Can you work these out from the model? Positions are in its coordinate system, mm. Coordinates: 2 decimals unless noted, no trailing zeros. Order: outer loops, then holes, each group sorted by start corner. A loop starts at its lowest first (then second) coordinate and runs counter-clockwise, first axis right, second up. Notation, with made-up numbers: (54, 1.5) -> (90, 1.5) arc R23 cw to (90, 38.5) -> close; hole circle Ø2 at (-13.5, 29.5). An arc over 180 degrees is marked (long way). Write item = value, one per line.
```python
from build123d import *

# Parameters (mm, degrees)
F0_R     = 14.732
F1_DEPTH = 3.175
F2_DEPTH = 2
F3_R     = 9.398
F4_DEPTH = 1.905
F6_R     = 0.635


# Not quite as in the source:
# - a fillet or chamfer that OpenCascade refuses, or shapes differently, is made with other operations: its cross-section is extruded or revolved along the edge and cut away or added


with BuildPart() as f1:
    # F0 (on Top) → F1 (new body)
    with BuildSketch(Plane.XY):
        Circle(F0_R)
        with BuildLine():
            ThreePointArc((-10.3772609868, 7.5395214312), (-6.4135, 11.1085078543), (-1.3407865983, 12.7567323519))
            Line((-1.3407865983, 12.7567323519), (-1.214689647, 11.557))
            Line((-1.214689647, 11.557), (1.214689647, 11.557))
            Line((1.214689647, 11.557), (1.3407865983, 12.7567323519))
            ThreePointArc((1.3407865983, 12.7567323519), (6.4135, 11.1085078543), (10.3772609868, 7.5395214312))
            Line((10.3772609868, 7.5395214312), (9.4013107681, 6.830452092))
            Line((9.4013107681, 6.830452092), (10.616000415, 4.726547908))
            Line((10.616000415, 4.726547908), (11.7180475852, 5.2172109207))
            ThreePointArc((11.7180475852, 5.2172109207), (12.827, 0), (11.7180475852, -5.2172109207))
            Line((11.7180475852, -5.2172109207), (10.616000415, -4.726547908))
            Line((10.616000415, -4.726547908), (9.4013107681, -6.830452092))
            Line((9.4013107681, -6.830452092), (10.3772609868, -7.5395214312))
            ThreePointArc((10.3772609868, -7.5395214312), (6.4135, -11.1085078543), (1.3407865983, -12.7567323519))
            Line((1.3407865983, -12.7567323519), (1.214689647, -11.557))
            Line((1.214689647, -11.557), (-1.214689647, -11.557))
            Line((-1.214689647, -11.557), (-1.3407865983, -12.7567323519))
            ThreePointArc((-1.3407865983, -12.7567323519), (-6.4135, -11.1085078543), (-10.3772609868, -7.5395214312))
            Line((-10.3772609868, -7.5395214312), (-9.4013107681, -6.830452092))
            Line((-9.4013107681, -6.830452092), (-10.616000415, -4.726547908))
            Line((-10.616000415, -4.726547908), (-11.7180475852, -5.2172109207))
            ThreePointArc((-11.7180475852, -5.2172109207), (-12.827, 0), (-11.7180475852, 5.2172109207))
            Line((-11.7180475852, 5.2172109207), (-10.616000415, 4.726547908))
            Line((-10.616000415, 4.726547908), (-9.4013107681, 6.830452092))
            Line((-9.4013107681, 6.830452092), (-10.3772609868, 7.5395214312))
        make_face(mode=Mode.SUBTRACT)
        with BuildLine():
            Line((-1.214689647, 11.557), (-1.3407865983, 12.7567323519))
            ThreePointArc((-1.3407865983, 12.7567323519), (-6.4135, 11.1085078543), (-10.3772609868, 7.5395214312))
            Line((-10.3772609868, 7.5395214312), (-9.4013107681, 6.830452092))
            Line((-9.4013107681, 6.830452092), (-10.616000415, 4.726547908))
            Line((-10.616000415, 4.726547908), (-11.7180475852, 5.2172109207))
            ThreePointArc((-11.7180475852, 5.2172109207), (-12.827, 0), (-11.7180475852, -5.2172109207))
            Line((-11.7180475852, -5.2172109207), (-10.616000415, -4.726547908))
            Line((-10.616000415, -4.726547908), (-9.4013107681, -6.830452092))
            Line((-9.4013107681, -6.830452092), (-10.3772609868, -7.5395214312))
            ThreePointArc((-10.3772609868, -7.5395214312), (-6.4135, -11.1085078543), (-1.3407865983, -12.7567323519))
            Line((-1.3407865983, -12.7567323519), (-1.214689647, -11.557))
            Line((-1.214689647, -11.557), (1.214689647, -11.557))
            Line((1.214689647, -11.557), (1.3407865983, -12.7567323519))
            ThreePointArc((1.3407865983, -12.7567323519), (6.4135, -11.1085078543), (10.3772609868, -7.5395214312))
            Line((10.3772609868, -7.5395214312), (9.4013107681, -6.830452092))
            Line((9.4013107681, -6.830452092), (10.616000415, -4.726547908))
            Line((10.616000415, -4.726547908), (11.7180475852, -5.2172109207))
            ThreePointArc((11.7180475852, -5.2172109207), (12.827, 0), (11.7180475852, 5.2172109207))
            Line((11.7180475852, 5.2172109207), (10.616000415, 4.726547908))
            Line((10.616000415, 4.726547908), (9.4013107681, 6.830452092))
            Line((9.4013107681, 6.830452092), (10.3772609868, 7.5395214312))
            ThreePointArc((10.3772609868, 7.5395214312), (6.4135, 11.1085078543), (1.3407865983, 12.7567323519))
            Line((1.3407865983, 12.7567323519), (1.214689647, 11.557))
            Line((1.214689647, 11.557), (-1.214689647, 11.557))
        make_face()
    extrude(amount=-F1_DEPTH)

    # F0 (on Top) → F2 (join)
    with BuildSketch(Plane.XY):
        Circle(F0_R)
        with BuildLine():
            ThreePointArc((-10.3772609868, 7.5395214312), (-6.4135, 11.1085078543), (-1.3407865983, 12.7567323519))
            Line((-1.3407865983, 12.7567323519), (-1.214689647, 11.557))
            Line((-1.214689647, 11.557), (1.214689647, 11.557))
            Line((1.214689647, 11.557), (1.3407865983, 12.7567323519))
            ThreePointArc((1.3407865983, 12.7567323519), (6.4135, 11.1085078543), (10.3772609868, 7.5395214312))
            Line((10.3772609868, 7.5395214312), (9.4013107681, 6.830452092))
            Line((9.4013107681, 6.830452092), (10.616000415, 4.726547908))
            Line((10.616000415, 4.726547908), (11.7180475852, 5.2172109207))
            ThreePointArc((11.7180475852, 5.2172109207), (12.827, 0), (11.7180475852, -5.2172109207))
            Line((11.7180475852, -5.2172109207), (10.616000415, -4.726547908))
            Line((10.616000415, -4.726547908), (9.4013107681, -6.830452092))
            Line((9.4013107681, -6.830452092), (10.3772609868, -7.5395214312))
            ThreePointArc((10.3772609868, -7.5395214312), (6.4135, -11.1085078543), (1.3407865983, -12.7567323519))
            Line((1.3407865983, -12.7567323519), (1.214689647, -11.557))
            Line((1.214689647, -11.557), (-1.214689647, -11.557))
            Line((-1.214689647, -11.557), (-1.3407865983, -12.7567323519))
            ThreePointArc((-1.3407865983, -12.7567323519), (-6.4135, -11.1085078543), (-10.3772609868, -7.5395214312))
            Line((-10.3772609868, -7.5395214312), (-9.4013107681, -6.830452092))
            Line((-9.4013107681, -6.830452092), (-10.616000415, -4.726547908))
            Line((-10.616000415, -4.726547908), (-11.7180475852, -5.2172109207))
            ThreePointArc((-11.7180475852, -5.2172109207), (-12.827, 0), (-11.7180475852, 5.2172109207))
            Line((-11.7180475852, 5.2172109207), (-10.616000415, 4.726547908))
            Line((-10.616000415, 4.726547908), (-9.4013107681, 6.830452092))
            Line((-9.4013107681, 6.830452092), (-10.3772609868, 7.5395214312))
        make_face(mode=Mode.SUBTRACT)
    extrude(amount=F2_DEPTH)

    # F3 (on face) → F4 (cut)
    with BuildSketch(Plane.XY):
        Circle(F3_R)
    extrude(amount=-F4_DEPTH, mode=Mode.SUBTRACT)

    # F5: fillet of radius 3.175 on 1 edges, made by hand

    # F5_s1 → F5_t2 (revolve, cut)
    with BuildSketch(Plane.XZ):
        with BuildLine():
            ThreePointArc((14.732, 0), (13.8020640303, -2.2450640303), (11.557, -3.175))
            Line((11.557, -3.175), (14.732, -3.175))
            Line((14.732, -3.175), (14.732, 0))
        make_face()
    revolve(axis=Axis((0, 0, -3.175), (0, 0, 1)), mode=Mode.SUBTRACT)

    # F6
    f6_edges = [f1.edges().sort_by_distance(p)[0] for p in [
        (0, 11.557, 2),
        (10.008656, -5.7785, 2),
        (-10.008656, 5.7785, 2),
        (-10.008656, -5.7785, 2),
        (0, -11.557, 2),
        (10.008656, 5.7785, 2),
    ]]
    fillet(f6_edges, radius=F6_R)


solid = f1.part
```
Item 1: I want a section at B-B, the plane y = 0. Please give me the cut outline in (x, z) (3 decimals), plus the area to 3 significant figures.
A:
outline = (-14.732, 0) arc R3.175 ccw to (-11.557, -3.175) -> (11.557, -3.175) arc R3.175 ccw to (14.732, 0) -> (14.732, 2) -> (12.827, 2) -> (12.827, 0) -> (9.398, 0) -> (9.398, -1.905) -> (-9.398, -1.905) -> (-9.398, 0) -> (-12.827, 0) -> (-12.827, 2) -> (-14.732, 2) -> close
area = 61.0 mm2
Item 2: I want a section at A-A, the plane x = 0. Please give me the cut outline in (y, z) (3 decimals).
A:
outline = (-14.732, 0) arc R3.175 ccw to (-11.557, -3.175) -> (11.557, -3.175) arc R3.175 ccw to (14.732, 0) -> (14.732, 2) -> (12.192, 2) arc R0.635 ccw to (11.557, 1.365) -> (11.557, 0) -> (9.398, 0) -> (9.398, -1.905) -> (-9.398, -1.905) -> (-9.398, 0) -> (-11.557, 0) -> (-11.557, 1.365) arc R0.635 ccw to (-12.192, 2) -> (-14.732, 2) -> close
Item 3: If I drill on probe 1 along Z at (x, y) = (-3, 5.75) (3 decimals); probe 2 along Z at (x, y) = (4, -9) (3 decimals); probe 3 along Y at (x, z) = (7.75, -0.3), over which ranges is the centre line in solid material (lowest first)?
A:
probe_1 = -3.175 to -1.905
probe_2 = -3.175 to 0
probe_3 = -12.51 to -5.32, 5.32 to 12.51
Item 4: If we mould it in two halves opening along Y, with no side actions, what happens to faces 1 (the flat face through (-11.16, -4.97, 0.99)), 2 (the flat face through (0, 0, -3.175))? For each: pulls with the +Y half, pulls with the -Y half, needs draft (parallel to the pull), parting line crosses it, or undercut.
A:
face_1 = undercut
face_2 = needs draft
Item 5: I want a section at C-C, the plane z = -1.5. Please give me the cut outline in (x, y).
A:
outline = circle Ø28.71 at (0, 0); hole circle Ø18.8 at (0, 0)
Item 6: I'm going to push flat-ended pins straight in: P1, Ø3, axis at x = 8, y = -8.5, coming from the +Z side; P2, Ø15, axis at x = 4.5, y = -1, coming from the +Z side; P3, Ø1, axis at y = -10, z = 0, coming from the -X side; P4, Ø1.5, axis at x = 0.5, y = -8, coming from the +Z side (3 decimals). Where does each tip first touch, or does it pass through?
A:
P1 = 2
P2 = 1.93
P3 = -11.26
P4 = -1.905
